Geometry check sheet. Reference: the model listing, model coordinates, mm. Give positions to 0.01 mm unless a question says otherwise; leave off trailing zeros. Write each loop counter-clockwise with the first axis right and the second up, starting at its lowest first coordinate (ties: lowest second). Pieces come first, ordered by that corner, then holes. Notation, with made-up numbers: (20.25, 83) - (43.25, 83) arc R27 cw to (43.25, 115) - close; hole circle Ø8 at (-27.75, -1). An arc over 180 degrees is marked (long way). Write item = value, one per line. Start each with the question number.
(1) Section check C-C, the plane y = 1. Give the number of separate pieces and of enclosed holes in the cut face, plus the area to 3 significant figures.
(2) Depth check by flat-ended pin: pin 1 Ø6 at (x, z) = (210, -40) entering from -Y; pin 2 Ø1.2 at (y, z) = (1.5, -230.5) entering from +X; pin 3 Ø1.2 at (x, y) = (63.5, 3) entering from -Z; pin 4 Ø2 at (x, y) = (238.5, 1.5) entering from +Z. Enter the tip coordinate at first touch or a pass-through.
(3) Draft check along Y on faces 1 (the flat face through (207, 4, -127)), 2 (the flat face through (207, 0, -127)). Enter one of: pulls with the +Y half, pulls with the -Y half, needs draft (parallel to the pull), parting line crosses it, or undercut.
(4) Section check A-A, the plane x = 194. Enter the section's corners in (y, z), plus the area to 3 significant figures.
(5) Section check B-B, the plane z = -91. Enter the section's corners in (x, y), plus the area to 3 significant figures.
(6) Thickness scan on L1, parallel to Z at x = 125, y = 2.35; L2, parallel to X at y = 2.7, z = -230; L3, parallel to X at y = 1.7, z = -115. Record the ranges inside material, lowest first.
```python
from build123d import *

# Parameters (mm, degrees)
CROQUIS1_W              = 250
CROQUIS1_H              = 250
CROQUIS1_R              = 2.5
SALIENTE_EXTRUIR1_DEPTH = 4
CORTAR_EXTRUIR1_DEPTH   = 4
CROQUIS3_W              = 150
CROQUIS3_H              = 150
CROQUIS3_W_2            = 100
CROQUIS3_H_2            = 100
SALIENTE_EXTRUIR2_DEPTH = 4
CROQUIS4_R              = 1.55
CORTAR_EXTRUIR2_DEPTH   = 10
CROQUIS5_W              = 150
CROQUIS5_H              = 150
CROQUIS5_W_2            = 100
CROQUIS5_H_2            = 100
CORTAR_EXTRUIR3_DEPTH   = 10
CROQUIS6_W              = 30
CROQUIS6_H              = 50
CROQUIS6_W_2            = 50
CROQUIS6_H_2            = 30
CORTAR_EXTRUIR4_DEPTH   = 10
CROQUIS8_R              = 1.55
CORTAR_EXTRUIR5_DEPTH   = 10


with BuildPart() as part:
    # Croquis1 → Saliente-Extruir1 (new body)
    with BuildSketch(Plane(origin=(0, 0, 0), x_dir=(1, 0, 0), z_dir=(0, 1, 0))):
        with Locations((125, 125)):
            Rectangle(CROQUIS1_W, CROQUIS1_H)
        with Locations(Location((40, 210, 0), (0, 0, 270))):
            Circle(CROQUIS1_R, mode=Mode.SUBTRACT)
        with Locations(Location((210, 210, 0), (0, 0, 270))):
            Circle(CROQUIS1_R, mode=Mode.SUBTRACT)
        with Locations(Location((210, 40, 0), (0, 0, 270))):
            Circle(CROQUIS1_R, mode=Mode.SUBTRACT)
        with Locations(Location((40, 40, 0), (0, 0, 270))):
            Circle(CROQUIS1_R, mode=Mode.SUBTRACT)
    extrude(amount=SALIENTE_EXTRUIR1_DEPTH)

    # Croquis2 → Cortar-Extruir1 (cut)
    with BuildSketch(Plane(origin=(0, 4, 0), x_dir=(1, 0, 0), z_dir=(0, 1, 0))):
        Polygon((50, 50), (200, 50), (200, 200), (50, 200), (50, 150.09044268), align=None)
    extrude(amount=-CORTAR_EXTRUIR1_DEPTH, mode=Mode.SUBTRACT)

    # Croquis3 → Saliente-Extruir2 (add)
    with BuildSketch(Plane(origin=(0, 4, 0), x_dir=(1, 0, 0), z_dir=(0, 1, 0))):
        with Locations((125, 125)):
            Rectangle(CROQUIS3_W, CROQUIS3_H)
        with Locations((125, 125)):
            Rectangle(CROQUIS3_W_2, CROQUIS3_H_2, mode=Mode.SUBTRACT)
    extrude(amount=-SALIENTE_EXTRUIR2_DEPTH)

    # Croquis4 → Cortar-Extruir2 (cut)
    with BuildSketch(Plane(origin=(0, 4, 0), x_dir=(1, 0, 0), z_dir=(0, 1, 0))):
        with Locations(Location((115, 20, 0), (0, 0, 270))):
            Circle(CROQUIS4_R)
        with Locations(Location((135, 20, 0), (0, 0, 270))):
            Circle(CROQUIS4_R)
        with Locations(Location((125, 5, 0), (0, 0, 270))):
            Circle(CROQUIS4_R)
    extrude(amount=-CORTAR_EXTRUIR2_DEPTH, mode=Mode.SUBTRACT)

    # Croquis5 → Cortar-Extruir3 (cut)
    with BuildSketch(Plane(origin=(0, 4, 0), x_dir=(1, 0, 0), z_dir=(0, 1, 0))):
        with Locations((125, 125)):
            Rectangle(CROQUIS5_W, CROQUIS5_H)
        with Locations((125, 125)):
            Rectangle(CROQUIS5_W_2, CROQUIS5_H_2, mode=Mode.SUBTRACT)
    extrude(amount=-CORTAR_EXTRUIR3_DEPTH, mode=Mode.SUBTRACT)

    # Croquis6 → Cortar-Extruir4 (cut)
    with BuildSketch(Plane(origin=(0, 4, 0), x_dir=(1, 0, 0), z_dir=(0, 1, 0))):
        Polygon((170, 0), (250, 0), (250, 30), (220, 30), (170, 30), align=None)
        with Locations((235, 55)):
            Rectangle(CROQUIS6_W, CROQUIS6_H)
        Polygon((0, 80), (0, 0), (30, 0), (30, 30), (30, 80), align=None)
        with Locations((55, 15)):
            Rectangle(CROQUIS6_W_2, CROQUIS6_H_2)
        Polygon((80, 250), (0, 250), (0, 220), (30, 220), (80, 220), align=None)
        with Locations((15, 195)):
            Rectangle(CROQUIS6_W, CROQUIS6_H)
        Polygon((250, 170), (250, 250), (220, 250), (220, 220), (220, 170), align=None)
        with Locations((195, 235)):
            Rectangle(CROQUIS6_W_2, CROQUIS6_H_2)
    extrude(amount=-CORTAR_EXTRUIR4_DEPTH, mode=Mode.SUBTRACT)

    # Croquis8 → Cortar-Extruir5 (cut)
    with BuildSketch(Plane(origin=(0, 4, 0), x_dir=(1, 0, 0), z_dir=(0, 1, 0))):
        with Locations(Location((125, 5, 0), (0, 0, 270))):
            Circle(CROQUIS8_R)
        with Locations(Location((135, 20, 0), (0, 0, 270))):
            Circle(CROQUIS8_R)
        with Locations(Location((115, 20, 0), (0, 0, 270))):
            Circle(CROQUIS8_R)
        with Locations(Location((20, 135, 0), (0, 0, 270))):
            Circle(CROQUIS8_R)
        with Locations(Location((5, 125, 0), (0, 0, 270))):
            Circle(CROQUIS8_R)
        with Locations(Location((20, 115, 0), (0, 0, 270))):
            Circle(CROQUIS8_R)
        with Locations(Location((135, 230, 0), (0, 0, 270))):
            Circle(CROQUIS8_R)
        with Locations(Location((125, 245, 0), (0, 0, 270))):
            Circle(CROQUIS8_R)
        with Locations(Location((115, 230, 0), (0, 0, 270))):
            Circle(CROQUIS8_R)
        with Locations(Location((230, 115, 0), (0, 0, 270))):
            Circle(CROQUIS8_R)
        with Locations(Location((245, 125, 0), (0, 0, 270))):
            Circle(CROQUIS8_R)
        with Locations(Location((230, 135, 0), (0, 0, 270))):
            Circle(CROQUIS8_R)
    extrude(amount=-CORTAR_EXTRUIR5_DEPTH, mode=Mode.SUBTRACT)


solid = part.part
```
Model answer:
q1.separate_pieces = 1
q1.enclosed_holes = 17
q1.area = 24,200 mm²
q2.pin_1 = 0
q2.pin_2 = 170
q2.pin_3 = -220
q2.pin_4 = -80
q3.face_1 = pulls with the +Y half
q3.face_2 = pulls with the -Y half
q4.outline = (0, -220) - (4, -220) - (4, -200) - (0, -200) - close; (0, -50) - (4, -50) - (4, -30) - (0, -30) - close
q4.area = 160 mm²
q5.outline = (0, 0) - (50, 0) - (50, 4) - (0, 4) - close; (200, 0) - (250, 0) - (250, 4) - (200, 4) - close
q5.area = 400 mm²
q6.L1 = -250 to -246.55, -243.45 to -200, -50 to -6.55, -3.45 to 0
q6.L2 = 80 to 113.45, 116.55 to 133.45, 136.55 to 170
q6.L3 = 0 to 18.45, 21.55 to 50, 200 to 228.45, 231.55 to 250
